from build123d import *

# Parameters (mm, degrees)
SKETCH_W        = 68
SKETCH_H        = 36
PAD_DEPTH       = 28
POCKET_DEPTH    = 20
SKETCH002_R     = 2.75
POCKET001_DEPTH = 28
POCKET002_DEPTH = 20


with BuildPart() as part:
    # Sketch → Pad (new body)
    with BuildSketch(Plane.XY):
        with Locations((34, 0)):
            Rectangle(SKETCH_W, SKETCH_H)
    extrude(amount=PAD_DEPTH)

    # Sketch001 (on DatumPlane) → Pocket (cut)
    with BuildSketch(Plane.XY.offset(28)):
        with BuildLine():
            Line((68, 10), (68, -10))
            Line((9, -10), (68, -10))
            ThreePointArc((8, -9), (7.292893, -10.707107), (9, -10))
            Line((8, 9), (8, -9))
            ThreePointArc((9, 10), (7.292893, 10.707107), (8, 9))
            Line((68, 10), (9, 10))
        make_face()
    extrude(amount=-POCKET_DEPTH, mode=Mode.SUBTRACT)

    # Sketch002 (on DatumPlane) → Pocket001 (cut)
    with BuildSketch(Plane.XY.offset(28)):
        with Locations((18, 0)):
            Circle(SKETCH002_R)
        with Locations((38, 0)):
            Circle(SKETCH002_R)
        with Locations((58, 0)):
            Circle(SKETCH002_R)
        with Locations((78, 0)):
            Circle(SKETCH002_R)
        with Locations((98, 0)):
            Circle(SKETCH002_R)
    extrude(amount=-POCKET001_DEPTH, mode=Mode.SUBTRACT)

    # Sketch003 (on DatumPlane) → Pocket002 (cut)
    with BuildSketch(Plane.XZ.offset(10)):
        Polygon((8, 8), (8, 10), (6, 8), align=None)
    extrude(amount=-POCKET002_DEPTH, mode=Mode.SUBTRACT)


solid = part.part
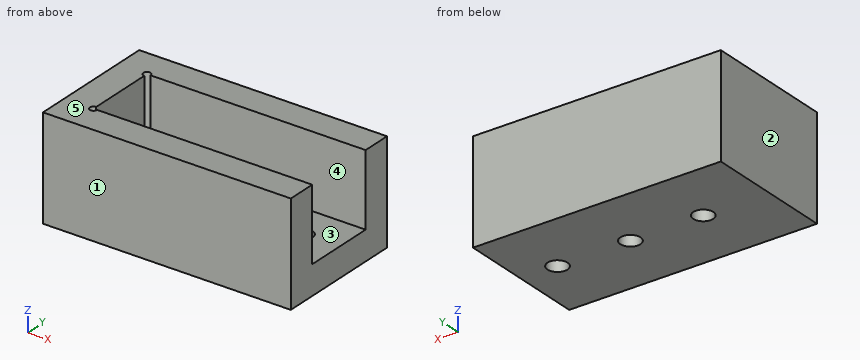
Design review of the part built by this model. Coordinates are the model's own, in mm. Face numbers are marked on the shaded views. A direction names the side the tool comes from. Coordinates: 2 decimals unless noted, no trailing zeros. Write each loop counter-clockwise with the first axis right and the second up, starting at its lowest first coordinate (ties: lowest second). Pieces come first, ordered by that corner, then holes. Notation, with made-up numbers: (82.5, -10.5) -> (93.5, -10.5) arc R24 ccw to (93.5, 6.5) -> close; hole circle Ø3 at (-1, 32.25). An arc over 180 degrees is marked (long way). Write each question's results on one line, items separated by ' | '. Start each with the question number.
(1) The part is to be moulded in two halves that separate along Y. For the marked faces 1, 2 and 3, say which applies: pulls with the +Y half, pulls with the -Y half, needs draft (parallel to the pull), parting line crosses it, or undercut.
(2) Clearance check with flat-ended pins moving along their axes: P1, Ø14.5, axis at y = -0.5, z = 17.5, coming from the +X side; P2, Ø7, axis at x = 38, y = 0, coming from the +Z side. State where each tip first meets the part, or that it passes through.
(3) Take a section at B-B on z = 5.5. Write out the cut boundary in (x, y), and give its area (3 significant figures).
(4) Tool access review of the marked faces 4 and 5: name each direction out of +Z, -Z, +X, -X, +Y, -Y from which nothing blocks a thin tool from reaching the whole face with its end or side.
(5) For line 1 along Y through (x, z) = (25.5, 17.25); line 2 along Y through (x, z) = (58, 3.25); line 3 along Z through (x, y) = (24.5, -6), list the stretches that pass through material, from the lowest coordinate up. Write a range as from..to.
(6) Take a section at C-C on x = 34. Write out the cut boundary in (y, z), and give its area (3 significant figures).
(7) Take a section at D-D on y = -6. Write out the cut boundary in (x, z), and give its area (3 significant figures).
(8) Take a section at A-A on y = 0. Write out the cut boundary in (x, z), and give its area (3 significant figures).
Results found:
1) face 1: pulls with the -Y half | face 2: needs draft | face 3: undercut
2) P1: stops at x = 8 | P2: stops at z = 8
3) outline: (0, -18) -> (68, -18) -> (68, 18) -> (0, 18) -> close; hole circle Ø5.5 at (18, 0); hole circle Ø5.5 at (38, 0); hole circle Ø5.5 at (58, 0) | area: 2,380 mm2
4) face 4: +Z, +X | face 5: +Z, +X, -X, +Y, -Y
5) line 1: y = -18..-10, 10..18 | line 2: y = -18..-2.75, 2.75..18 | line 3: z = 0..8
6) outline: (-18, 0) -> (18, 0) -> (18, 28) -> (10, 28) -> (10, 8) -> (-10, 8) -> (-10, 28) -> (-18, 28) -> close | area: 608 mm2
7) outline: (0, 0) -> (68, 0) -> (68, 8) -> (6, 8) -> (8, 10) -> (8, 28) -> (0, 28) -> close | area: 702 mm2
8) outline: (0, 0) -> (15.25, 0) -> (15.25, 8) -> (6, 8) -> (8, 10) -> (8, 28) -> (0, 28) -> close; (20.75, 0) -> (35.25, 0) -> (35.25, 8) -> (20.75, 8) -> close; (40.75, 0) -> (55.25, 0) -> (55.25, 8) -> (40.75, 8) -> close; (60.75, 0) -> (68, 0) -> (68, 8) -> (60.75, 8) -> close | area: 570 mm2
